Geometry check sheet. Reference: the model listing, model coordinates, mm. Coordinates: 2 decimals unless noted, no trailing zeros. Order: outer loops, then holes, each group sorted by start corner. A loop starts at its lowest first (then second) coordinate and runs counter-clockwise, first axis right, second up. Notation, with made-up numbers: M 66,-0.5 L 79,-0.5 A21 cw 79,17.5 Z; hole C 78,55 d9. An arc over 180 degrees is marked long. One line per item, written item: value. Start each with the question number.
1) Sectioned sample at C-C, the plane y = 9.75. State how many separate pieces and enclosed holes the cut face has, then the cut area to 3 significant figures.
2) Go/stop test with flat-tipped pins: P1, Ø5.5, axis at x = 218.5, z = -190.21, coming from the -Y side; P2, Ø4, axis at x = 104.5, y = 10.5, coming from the -Z side; P3, Ø2, axis at y = 10.5, z = -200.5, coming from the -X side; P4, Ø5, axis at x = 50.5, y = 4.5, coming from the -Z side. Record where each tip stops, or that it passes through.
3) Sectioned sample at B-B, the plane x = 172.5. Enter the section's corners in (y, z).
4) Thickness scan on L1, parallel to X at y = 3.5, z = 0; L2, parallel to X at y = 1.5, z = 188.5; L3, parallel to Z at x = 4, y = 9.5. Record the ranges inside material, lowest first. Write a range as from..to.
5) Sectioned sample at A-A, the plane z = 0. Enter the section's corners in (x, y).
6) Draft check along X on faces 1 (the cylindrical face through (11.13, 5.916, -253.756)), 2 (the cylindrical face through (13.768, 5.916, -313.698)), 3 (the flat face through (1, 12, -257)). Enter one of: pulls with the +X half, pulls with the -X half, needs draft (parallel to the pull), parting line crosses it, or undercut.
```python
from build123d import *

# Parameters (mm, degrees)
SKETCH1_R           = 314
SKETCH1_R_2         = 254
BOSS_EXTRUDE1_DEPTH = 12
SKETCH2_W           = 5.489817528
SKETCH2_H           = 110.495913403
CUT_EXTRUDE1_DEPTH  = 445.22516813
SKETCH3_R           = 3.45
SCREW_HOLE_DEPTH    = 445.22516813
CIRPATTERN1_COUNT   = 4


with BuildPart() as part:
    # Sketch1 → Boss-Extrude1 (new body)
    with BuildSketch(Plane(origin=(0, 0, 0), x_dir=(1, 0, 0), z_dir=(0, 1, 0))):
        with Locations(Location((0, 0, 0), (0, 0, 270))):
            Circle(SKETCH1_R)
        with Locations(Location((0, 0, 0), (0, 0, 270))):
            Circle(SKETCH1_R_2, mode=Mode.SUBTRACT)
    extrude(amount=BOSS_EXTRUDE1_DEPTH)

    # Sketch2 → Cut-Extrude1 (cut, through all)
    with BuildSketch(Plane(origin=(0, 12, 0), x_dir=(1, 0, 0), z_dir=(0, 1, 0))):
        with Locations((0, -289.886753328)):
            Rectangle(SKETCH2_W, SKETCH2_H)
    extrude(amount=-CUT_EXTRUDE1_DEPTH, mode=Mode.SUBTRACT)

    # Sketch3 → screw hole (cut, through all)
    with BuildSketch(Plane(origin=(0, 12, 0), x_dir=(1, 0, 0), z_dir=(0, 1, 0))):
        with Locations(Location((190.211724139, -218.495995387, 0), (0, 0, 270))):
            Circle(SKETCH3_R)
        with Locations(Location((218.495995387, -190.211724139, 0), (0, 0, 270))):
            Circle(SKETCH3_R)
    screw_hole = extrude(amount=-SCREW_HOLE_DEPTH, mode=Mode.SUBTRACT)

    # CirPattern1: screw hole ×4 about axis
    cirpattern1_axis = Axis((0, 0, 0), (0, 1, 0))
    for i in range(1, CIRPATTERN1_COUNT):
        add(screw_hole.rotate(cirpattern1_axis, i * 360 / CIRPATTERN1_COUNT), mode=Mode.SUBTRACT)


solid = part.part
```
Final values:
1. separate pieces: 1
1. enclosed holes: 8
1. area: 106,000 mm^2
2. P1: passes through
2. P2: stops at z = -296.8
2. P3: stops at x = -242.48
2. P4: stops at z = -310.31
3. outline: M 0,-262.37 L 12,-262.37 L 12,-186.44 L 0,-186.44 Z; M 0,186.44 L 12,186.44 L 12,262.37 L 0,262.37 Z
4. L1: x = -314..-254, 254..314
4. L2: x = -251.12..-221.49, -215.5..-170.25, 170.25..215.5, 221.49..251.12
4. L3: z = -313.97..-253.97, 253.97..313.97
5. outline: M -314,0 L -254,0 L -254,12 L -314,12 Z; M 254,0 L 314,0 L 314,12 L 254,12 Z
6. face 1: undercut
6. face 2: parting line crosses it
6. face 3: needs draft
